Read the model definition and answer for the solid it produces. Units are mm, in the model's axes. Face numbers are marked on the shaded views. A direction names the side the tool comes from. Coordinates: 2 decimals unless noted, no trailing zeros. Order: outer loops, then holes, each group sorted by start corner. A loop starts at its lowest first (then second) coordinate and runs counter-clockwise, first axis right, second up. Notation, with made-up numbers: (3, 28.5) -> (25, 28.5) arc R10 ccw to (25, 45.5) -> close; hole circle Ø2 at (25, 73.5). An arc over 180 degrees is marked (long way). Answer in a Markdown table with one row per item.
Autodesk Inventor part; units mm, degrees
ref_plane "YZ Plane" through (0, 0, 0) normal (1, 0, 0) x (0, 1, 0)
ref_plane "XZ Plane" through (0, 0, 0) normal (0, 1, 0) x (-1, 0, 0)
ref_plane "XY Plane" through (0, 0, 0) normal (0, 0, 1) x (1, 0, 0)
sketch "Sketch1" plane through (0, 0, 0) normal (0, 1, 0) x (-1, 0, 0)
  line L0 (0, 0) -> (0, -50.8)
  line L1 (0, -50.8) -> (50.8, 0)
  line L2 (50.8, 0) -> (0, 0)
  dimension "d0" = 50.8
extrude "Extrusion1" add sketch "Sketch1" along normal blind 12.7
shell "Shell1" thickness 3.175 removed faces 2 at (-16.9333, 8.4667, -33.8667) at (-16.9333, 12.7, -16.9333)
properties part number "Corner_Brace"
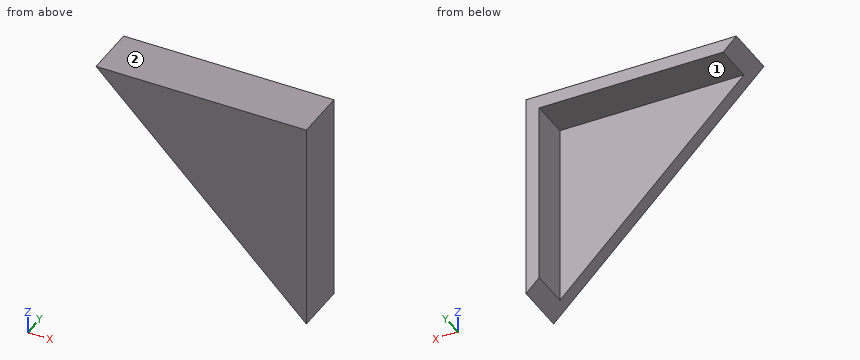
Q1. For the marked faces 1 and 2, determine the directions among +Z, -Z, +X, -X, +Y, -Y from which every point of the face is accessible in a straight line to the end or side of a thin tool.
Outcome:
| item | result |
|---|---|
| face 1 | -Z, -X, +Y |
| face 2 | +Z, +X, -X, +Y, -Y |
Q2. The part is cut by section A-A (x = -21.5). Write down the section's boundary in (y, z) (3 decimals).
Outcome:
| item | result |
|---|---|
| outline | (0, -29.3) -> (3.175, -29.3) -> (3.175, -3.175) -> (12.7, -3.175) -> (12.7, 0) -> (0, 0) -> close |
Q3. The part is cut by section B-B (z = -44.5). Write down the section's boundary in (x, y) (3 decimals), then the cut area to 3 significant figures.
Outcome:
| item | result |
|---|---|
| outline | (-6.3, 0) -> (0, 0) -> (0, 12.7) -> (-3.175, 12.7) -> (-3.175, 3.175) -> (-6.3, 3.175) -> close |
| area | 50.2 mm² |
Q4. Given pin 1 (5 mm diameter, centred on x = -22, y = 6.5, fed in from +Z); pin 2 (7.5 mm diameter, centred on x = -25, y = 7, fed in from -Z) (3 decimals); pin 3 (4 mm diameter, centred on y = 5.5, z = -11, fed in from -X) (3 decimals); pin 4 (2 mm diameter, centred on x = -7.5, z = -18.5, fed in from +Y) (3 decimals), each flat-ended and moving along its own axis, determine where each tip first touches the part or whether it passes through.
Outcome:
| item | result |
|---|---|
| pin 1 | z = 0 |
| pin 2 | z = -3.175 |
| pin 3 | x = -3.175 |
| pin 4 | y = 3.175 |
Q5. Consider line 1 (X direction, y = 11.25, z = -30) (3 decimals); line 2 (Y direction, x = -28, z = -10) (3 decimals). Determine where each line is inside the solid, lowest interval first.
Outcome:
| item | result |
|---|---|
| line 1 | -3.175 to 0 |
| line 2 | 0 to 3.175 |
Q6. The part is cut by section C-C (y = 1.5). Write down the section's boundary in (x, z), then the cut area to 3 significant figures.
Outcome:
| item | result |
|---|---|
| outline | (-50.8, 0) -> (0, -50.8) -> (0, 0) -> close |
| area | 1,290 mm² |
